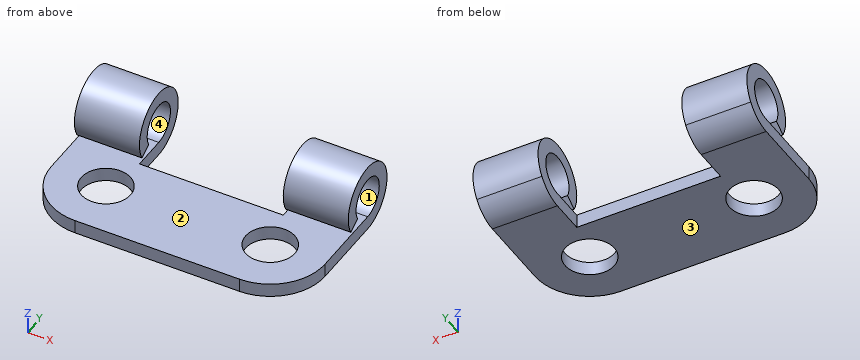
from build123d import *

# Parameters (mm, degrees)
SM_BASE_FLANGE_1_DEPTH = 1
OTHER_START            = -10
OTHER_1_DEPTH          = 20
OTHER_1_2_DEPTH        = 4.75
OTHER_START_2          = 5.25
OTHER_1_3_DEPTH        = 4.75
FILLET_1_R             = 4
HOLE_WIZARD_M31_D      = 3.6


# Read off the part's stored shape, not the designer's step: Каемка1
# Sheet-metal steps are written as plain solids
with BuildPart() as part:
    # Sketch 1 → Базовая кромка1 (new body)
    with BuildSketch(Plane.XY):
        Polygon((5.25, 6), (5.25, 1), (-5.25, 1), (-5.25, 6), (-10, 6), (-10, -6), (10, -6), (10, 6), align=None)
    extrude(amount=-SM_BASE_FLANGE_1_DEPTH)

    # Other 1 outline → Other 1 (cut)
    with BuildSketch(Plane.YZ.offset(OTHER_START)):
        with BuildLine():
            Line((6, 0), (5.5, 0))
            ThreePointArc((5.5, 0), (4.618033989, -0.736067978), (3.5, -1))
            Line((3.5, -1), (6, -1))
            Line((6, -1), (6, 0))
        make_face()
    extrude(amount=OTHER_1_DEPTH, mode=Mode.SUBTRACT)

    # Other 1 2 outline → Other 1 2 (add)
    with BuildSketch(Plane.YZ.offset(OTHER_START)):
        with BuildLine():
            Line((1.334936491, 0.25), (2.200961894, 0.75))
            ThreePointArc((2.200961894, 0.75), (4.25, 2.799038106), (3.5, 0))
            Line((3.5, 0), (5.5, 0))
            ThreePointArc((5.5, 0), (3.649788152, 3.995508667), (1.334936491, 0.25))
        make_face()
    extrude(amount=OTHER_1_2_DEPTH)

    # Other 1 3 outline → Other 1 3 (add)
    with BuildSketch(Plane.YZ.offset(OTHER_START_2)):
        with BuildLine():
            Line((1.334936491, 0.25), (2.200961894, 0.75))
            ThreePointArc((2.200961894, 0.75), (4.25, 2.799038106), (3.5, 0))
            Line((3.5, 0), (5.5, 0))
            ThreePointArc((5.5, 0), (3.649788152, 3.995508667), (1.334936491, 0.25))
        make_face()
    extrude(amount=OTHER_1_3_DEPTH)

    # Скругление1
    fillet_1_edges = [part.edges().sort_by_distance(p)[0] for p in [
        (10, -6, -0.5),
        (-10, -6, -0.5),
    ]]
    fillet(fillet_1_edges, radius=FILLET_1_R)

    # Отверстие с зазором M31 (through all)
    with Locations(Plane.XY):
        with Locations((6, -2), (-6, -2)):
            Hole(HOLE_WIZARD_M31_D / 2)


solid = part.part
Work out the finished part from the listing and answer in its coordinate system (mm). Face numbers are marked on the shaded views. A direction names the side the tool comes from. Give positions to 0.01 mm unless a question says otherwise; leave off trailing zeros. Loops run counter-clockwise (first coordinate to the right, second up) from the corner with the lowest first, then second, coordinate; pieces in that order, holes last. Notation, with made-up numbers: (56.25, 51.5) - (95.25, 51.5) arc R34 ccw to (95.25, 90.5) - close; hole circle Ø8 at (-38.5, 72). An arc over 180 degrees is marked (long way). Answer in a Markdown table with one row per item.
(1) Section B-B (x = 4.5) is taken. Give the vertices of the cut face in (y, z), and give its area (3 significant figures).
Results list:
| item | result |
|---|---|
| outline | (-6, -1) - (-2.99, -1) - (-2.99, 0) - (-6, 0) - close; (-1.01, -1) - (1, -1) - (1, 0) - (-1.01, 0) - close |
| area | 5.01 mm² |
(2) Section C-C (z = 3.25) is taken. Give the vertices of the cut face in (x, y), and give its area (3 significant figures).
Results list:
| item | result |
|---|---|
| outline | (-10, 1.71) - (-5.25, 1.71) - (-5.25, 5.29) - (-10, 5.29) - close; (5.25, 1.71) - (10, 1.71) - (10, 5.29) - (5.25, 5.29) - close |
| area | 33.9 mm² |
(3) Section D-D (x = -7.5) is taken. Give the vertices of the cut face in (y, z), and give its area (3 significant figures).
Results list:
| item | result |
|---|---|
| outline | (-5.71, -1) - (-2.99, -1) - (-2.99, 0) - (-5.71, 0) - close; (-1.01, -1) - (3.5, -1) arc R2.5 ccw (long way) to (1.33, 0.25) - (2.2, 0.75) arc R1.5 cw (long way) to (3.5, 0) - (-1.01, 0) - close |
| area | 17.7 mm² |
(4) Section A-A (z = 1.5) is taken. Give the vertices of the cut face in (x, y).
Results list:
| item | result |
|---|---|
| outline | (-10, 1) - (-5.25, 1) - (-5.25, 2) - (-10, 2) - close; (-10, 5) - (-5.25, 5) - (-5.25, 6) - (-10, 6) - close; (5.25, 1) - (10, 1) - (10, 2) - (5.25, 2) - close; (5.25, 5) - (10, 5) - (10, 6) - (5.25, 6) - close |
(5) A tool of negligible diameter and unlimited length cuts with its end or side. For the marked faces 1 and 2, from which of +Z, -Z, +X, -X, +Y, -Y can it reach the whole face along a straight path? Write none if from no direction.
Results list:
| item | result |
|---|---|
| face 1 | +X, -X |
| face 2 | +X, -X, -Y |
(6) Flat-ended cylindrical pins translate along their axes: pin 1 Ø4 at (x, y) = (-6, -2) entering from +Z; pin 2 Ø1.5 at (y, z) = (0.5, 3) entering from -X; pin 3 Ø0.8 at (x, z) = (-1, -0.5) entering from +Y; pin 4 Ø2 at (x, z) = (4.5, -0.5) entering from +Y. Find the tip coordinate at first contact, or state that the pin passes through.
Results list:
| item | result |
|---|---|
| pin 1 | stops at z = 0 |
| pin 2 | passes through |
| pin 3 | stops at y = 1 |
| pin 4 | stops at y = 5.61 |
(7) Consider L1, parallel to Y at x = 7.4, z = 1.5; L2, parallel to Z at x = 9, y = 3.5; L3, parallel to X at y = 1.5, z = 2. Determine where each line is inside the solid, lowest interval first. Write a range as [from, to].
Results list:
| item | result |
|---|---|
| L1 | y = [1, 2], [5, 6] |
| L2 | z = [-1, 0], [3, 4] |
| L3 | x = [-10, -5.25], [5.25, 10] |
(8) For a pull along Z with two mould halves and no side action, classify the marked faces 3 and 4 as pulls with the +Z half, pulls with the -Z half, needs draft (parallel to the pull), parting line crosses it, or undercut.
Results list:
| item | result |
|---|---|
| face 3 | pulls with the -Z half |
| face 4 | undercut |
